Autodesk Inventor part; units mm, degrees
ref_plane "YZ Plane" through (0, 0, 0) normal (1, 0, 0) x (0, 1, 0)
ref_plane "XZ Plane" through (0, 0, 0) normal (0, 1, 0) x (-1, 0, 0)
ref_plane "XY Plane" through (0, 0, 0) normal (0, 0, 1) x (1, 0, 0)
sketch "Sketch1" plane through (0, 0, 0) normal (0, 1, 0) x (-1, 0, 0)
  line L0 (0, 0) -> (-19, 0)
  line L1 (-19, 0) -> (-19, -41.2)
  line L2 (-19, -41.2) -> (0, -41.2)
  line L3 (0, -41.2) -> (0, 0)
  line L4 (-1.75, 0) -> (-1.75, -41.2)
  line L5 (0, -39.25) -> (-19, -39.25)
  circle A0 centre (-3.425, -3.525) radius 1.675
  circle A1 centre (-3.425, -37.575) radius 1.675
  line L6 (-8.7, -21.2) -> (-15.3, -21.2)
  line L7 (-15.3, -21.2) -> (-15.3, -32.5)
  line L8 (-15.3, -32.5) -> (-8.7, -32.5)
  line L9 (-8.7, -32.5) -> (-8.7, -21.2)
  line L10 (-7, -1.7) -> (-19.8, -1.7)
  line L11 (-19.8, -1.7) -> (-19.8, -13.3)
  line L12 (-19.8, -13.3) -> (-7, -13.3)
  line L13 (-7, -13.3) -> (-7, -1.7)
  line L14 (0, -1.85) -> (-19, -1.85)
  dimension "d0" = 19
  dimension "d1" = 41.2
  dimension "d2" = 1.75
  dimension "d4" = 1.95
  dimension "d5" = 3.35
  dimension "d6" = 3.35
  dimension "d7" = 6.6
  dimension "d8" = 11.3
  dimension "d11" = 8.7
  dimension "d12" = 8.7
  dimension "d13" = 12.8
  dimension "d14" = 11.6
  dimension "d16" = 1.7
  dimension "d27" = 1.85
  dimension "d28" = 7
extrude "Extrusion1" add sketch "Sketch1" along normal blind 0.8 contours L3 L14 L4 L0 | L4 L14 L13 L10 L1 L0 | L3 L5 L4 L14 | L4 A0 L14 | L3 L2 L4 L5 | L10 L13 L14 L1 | L4 A1 L5 L1 L12 L13 L14 A0 | L5 A1 L4 | L4 L2 L1 L5 | L14 L13 L12 L1 | L9 L8 L7 L6
extrude "Extrusion2" add sketch "Sketch1" along normal blind 5.2 contours L10 L13 L14 L1 | L1 L12 L11 L10 | L14 L13 L12 L1
extrude "Extrusion3" add sketch "Sketch1" along normal blind 4.5 contours L9 L8 L7 L6
chamfer "Chamfer1" distance 2 angle 45 2 edges at (15.3, 0.8, -26.85) (8.7, 0.8, -26.85)
sketch "Sketch2" plane through (0, 0, 0) normal (0, -1, 0) x (1, 0, 0)
  line L0 (19, 0) -> (19, -1.7)
  line L1 (0, 0) -> (19, 0)
  line L2 (0, -41.2) -> (0, 0)
  line L3 (19, -41.2) -> (0, -41.2)
  line L4 (19, -13.3) -> (19, -41.2)
  line L5 (19.8, -13.3) -> (19, -13.3)
  line L6 (19.8, -1.7) -> (19.8, -13.3)
  line L7 (19, -1.7) -> (19.8, -1.7)
  circle A0 centre (3.425, -3.525) radius 1.675
  circle A1 centre (3.425, -37.575) radius 1.675
  line L8 (0, -41.2) -> (19, -41.2)
  line L9 (19, -41.2) -> (19, 0)
  line L10 (19, 0) -> (0, 0)
  line L11 (0, 0) -> (0, -41.2)
  line L12 (6.4, 0) -> (16.8, 0)
  line L13 (16.8, 0) -> (16.8, -4.5)
  line L14 (16.8, -4.5) -> (6.4, -4.5)
  line L15 (6.4, -4.5) -> (6.4, 0)
  line L16 (9.8, -41.2) -> (16.8, -41.2)
  line L17 (16.8, -41.2) -> (16.8, -36.2)
  line L18 (16.8, -36.2) -> (9.8, -36.2)
  line L19 (9.8, -36.2) -> (9.8, -41.2)
  dimension "d29" = 10.4
  dimension "d30" = 4.5
  dimension "d31" = 0
  dimension "d32" = 6.4
  dimension "d33" = 7
  dimension "d34" = 5
  dimension "d35" = 2.2
  dimension "d36" = 0
extrude "Extrusion4" add sketch "Sketch2" along normal blind 3.5 contours L13 L14 L15 L1 | L3 L19 L18 L17
properties part number "interface_board"
Model file for the job. Use its own axes, mm. A direction names the side the tool comes from. Coordinates: 2 decimals unless noted, no trailing zeros. Write each loop counter-clockwise with the first axis right and the second up, starting at its lowest first coordinate (ties: lowest second). Pieces come first, ordered by that corner, then holes. Notation, with made-up numbers: (-14.5, -4) - (26.5, -4) arc R34 ccw to (26.5, 33) - close; hole circle Ø2 at (43, 67.5). An arc over 180 degrees is marked (long way). Use a Markdown table: item, result. Add a question column.
Item 1: Drop flat-ended pins along their axis: pin 1 (1 mm diameter, centred on y = -1, z = -30.5, fed in from -X); pin 2 (1.9 mm diameter, centred on y = 4, z = -24, fed in from -X); pin 3 (4 mm diameter, centred on x = 12, z = -13.5, fed in from +Y); pin 4 (1.4 mm diameter, centred on y = 4, z = -25, fed in from +X). Give the stop position or say it passes through.
Item 2: Band-saw the part on A-A, the plane y = 2. Write the cut outline in (x, z), and give its area (3 significant figures).
Item 3: Band-saw the part on D-D, the plane x = 14.75. Write the cut outline in (y, z), and give its area (3 significant figures).
Item 4: Band-saw the part on B-B, the plane z = -23.5. Write the cut outline in (x, y), and give its area (3 significant figures).
Item 5: Drill centre lines: line 1 along Z through (x, y) = (14, 1.5); line 2 along Z through (x, y) = (10.5, -0.75); line 3 along X through (y, z) = (3.5, -4). Where is each one in solid material? Low to high.
Item 6: Two-plate mould, pull along Z, no slides. Class faces 1 (the face through (13, -2, -36.2)), 2 (the face through (11, -1, 0)), 3 (the face through (9.8, -2, -39)): pulls with the +Z half, pulls with the -Z half, needs draft (parallel to the pull), parting line crosses it, or undercut.
Item 7: 3-axis set-ups, long thin cutter, end or side, ignore diameter. For faces 4 (the face through (7.7, 1.8, -26.9)), 5 (the face through (16.8, -2, -39)), 6 (the face through (16.3, 1.8, -26.8)): which of +Z, -Z, +X, -X, +Y, -Y reach the whole face in a straight line?
Item 8: Band-saw the part on C-C, the plane x = 3. Write the cut outline in (y, z).
A:
| question | item | result |
|---|---|---|
| 1 | pin 1 | passes through |
| 1 | pin 2 | stops at x = 8.7 |
| 1 | pin 3 | stops at y = 5.2 |
| 1 | pin 4 | stops at x = 15.3 |
| 2 | outline | (7, -13.3) - (19.8, -13.3) - (19.8, -1.7) - (7, -1.7) - close; (7.9, -32.5) - (16.1, -32.5) - (16.1, -21.2) - (7.9, -21.2) - close |
| 2 | area | 241 mm² |
| 3 | outline | (-3.5, -41.2) - (0.8, -41.2) - (0.8, -32.5) - (4.5, -32.5) - (4.5, -21.2) - (0.8, -21.2) - (0.8, -13.3) - (5.2, -13.3) - (5.2, -1.7) - (0.8, -1.7) - (0.8, 0) - (-3.5, 0) - (-3.5, -4.5) - (0, -4.5) - (0, -36.2) - (-3.5, -36.2) - close |
| 3 | area | 159 mm² |
| 4 | outline | (0, 0) - (19, 0) - (19, 0.8) - (17.3, 0.8) - (15.3, 2.8) - (15.3, 4.5) - (8.7, 4.5) - (8.7, 2.8) - (6.7, 0.8) - (0, 0.8) - close |
| 4 | area | 43.6 mm² |
| 5 | line 1 | z = -32.5 to -21.2, -13.3 to -1.7 |
| 5 | line 2 | z = -41.2 to -36.2, -4.5 to 0 |
| 5 | line 3 | x = 7 to 19.8 |
| 6 | face 1 | undercut |
| 6 | face 2 | pulls with the +Z half |
| 6 | face 3 | needs draft |
| 7 | face 4 | -Z, -X, +Y |
| 7 | face 5 | +Z, -Z, +X, -Y |
| 7 | face 6 | -Z, +X, +Y |
| 8 | outline | (0, -41.2) - (0.8, -41.2) - (0.8, -39.2) - (0, -39.2) - close; (0, -35.95) - (0.8, -35.95) - (0.8, -5.15) - (0, -5.15) - close; (0, -1.9) - (0.8, -1.9) - (0.8, 0) - (0, 0) - close |
